from build123d import *

# Parameters (mm, degrees)
SKETCH3_W           = 609.6
SKETCH3_H           = 304.8
BOSS_EXTRUDE1_DEPTH = 304.8
SKETCH4_W           = 609.6
SKETCH4_H           = 177.8
CUT_EXTRUDE1_DEPTH  = 609.6
SKETCH6_W           = 609.6
SKETCH6_H           = 609.6
CUT_EXTRUDE2_DEPTH  = 254


with BuildPart() as part:
    # Sketch3 → Boss-Extrude1 (new, symmetric)
    with BuildSketch(Plane.XY):
        Rectangle(SKETCH3_W, SKETCH3_H)
    extrude(amount=BOSS_EXTRUDE1_DEPTH, both=True)

    # Sketch4 → Cut-Extrude1 (cut)
    with BuildSketch(Plane(origin=(0, 0, -304.8), x_dir=(-1, 0, 0), z_dir=(0, 0, -1))):
        with Locations((0, -63.5)):
            Rectangle(SKETCH4_W, SKETCH4_H)
    extrude(amount=-CUT_EXTRUDE1_DEPTH, mode=Mode.SUBTRACT)

    # Sketch6 → Cut-Extrude2 (cut)
    with BuildSketch(Plane(origin=(0, 152.4, 0), x_dir=(1, 0, 0), z_dir=(0, 1, 0))):
        Rectangle(SKETCH6_W, SKETCH6_H)
        with BuildLine():
            Line((59.856357946, 27.628202152), (59.856357946, 30.803202152))
            ThreePointArc((59.856357946, 30.803202152), (-105.908299402, -7.521579235), (-239.166769949, -113.299131305))
            Line((-239.166769949, -113.299131305), (-235.991769949, -113.299131305))
            ThreePointArc((-235.991769949, -113.299131305), (-103.99313709, -9.40327752), (59.856357946, 27.628202152))
        make_face(mode=Mode.SUBTRACT)
    extrude(amount=-CUT_EXTRUDE2_DEPTH, mode=Mode.SUBTRACT)


solid = part.part
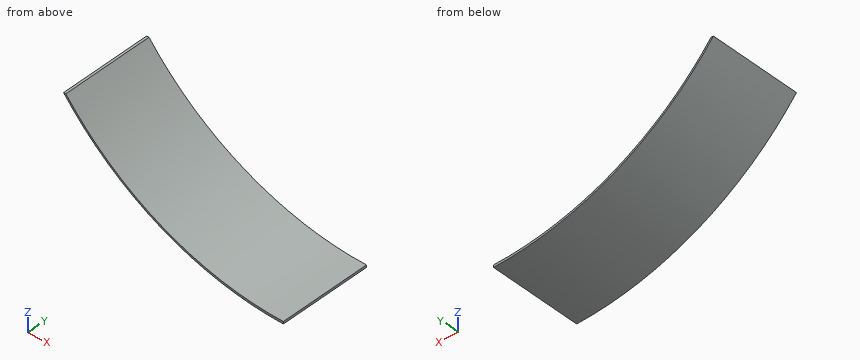
Verification items for the finished model (mm, model axes). Give positions to 0.01 mm unless a question says otherwise; leave off trailing zeros. Order: outer loops, then holes, each group sorted by start corner. A loop starts at its lowest first (then second) coordinate and runs counter-clockwise, first axis right, second up. Notation, with made-up numbers: M 28,29 L 68,29 A25 ccw 68,52 Z; hole C 9,-31.5 d4. An arc over 180 degrees is marked long. Use one line per item in the form item = value. Start each with the question number.
Q1. Scan lines: line 1 along X through (y, z) = (139, 38.5); line 2 along Z through (x, y) = (27, 31); line 3 along Z through (x, y) = (-89, 43.5). Record each from-to range of solid material in increasing order. Write a range as [from, to].
Q2. Section check B-B (x = -139). Enter the section's corners in (y, z), then the cut area to 3 significant figures.
Q3. Go/stop test with flat-tipped pins: pin 1 Ø1.5 at (y, z) = (93, 46) entering from +X; pin 2 Ø5 at (x, y) = (29, 120.5) entering from -Z; pin 3 Ø6 at (x, y) = (-47, 94.5) entering from -Z. Record where each tip stops, or that it passes through.
Q4. Section check A-A (y = 115). Enter the section's corners in (x, z).
Evaluation:
q1.line_1 = [-158.95, -154.66]
q1.line_2 = [-29.23, -26.21]
q1.line_3 = [-0.13, 2.65]
q2.outline = M 25.4,25.51 L 152.4,25.51 L 152.4,28.38 L 25.4,28.38 Z
q2.area = 366 mm2
q3.pin_1 = -164.25
q3.pin_2 = -29.61
q3.pin_3 = -16.01
q4.outline = M -239.17,113.3 A386.59 ccw 59.86,-30.8 L 59.86,-27.63 A381 cw -235.99,113.3 Z
